Here's how the part is built. I have some questions about the finished solid (model axes, mm). Face numbers are marked on the shaded views. A direction names the side the tool comes from. Give positions to 0.01 mm unless a question says otherwise; leave off trailing zeros. Write each loop counter-clockwise with the first axis right and the second up, starting at its lowest first coordinate (ties: lowest second). Pieces come first, ordered by that corner, then holes. Notation, with made-up numbers: (56.5, 49.5) -> (72.5, 49.5) arc R23 cw to (72.5, 60.5) -> close; hole circle Ø5 at (88, 48.5). An arc over 180 degrees is marked (long way). Use one line per item in the form item = value.
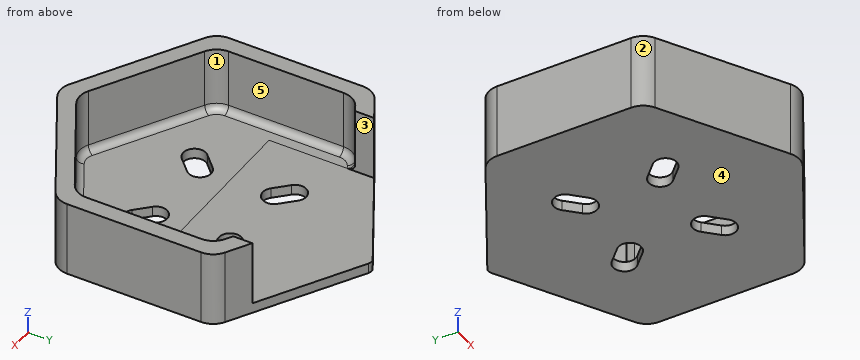
```python
from build123d import *

# Parameters (mm, degrees)
F1_DEPTH = 1.5
F2_DEPTH = 11
F4_W     = 30
F4_H     = 11.070783
F5_DEPTH = 26
F6_R     = 3
F7_R     = 1


with BuildPart() as f1:
    # F0 (on Top) → F1 (new body)
    with BuildSketch(Plane.XY):
        Polygon((0, -20.207259), (17.5, -10.10363), (17.5, 10.10363), (0, 20.207259), (-17.5, 10.10363), (-17.5, -10.10363), align=None)
        with BuildLine():
            ThreePointArc((-6.151829, -8.485281), (-8.485281, -8.485281), (-8.485281, -6.151829))
            Line((-8.485281, -6.151829), (-6.576093, -4.242641))
            ThreePointArc((-6.576093, -4.242641), (-4.242641, -4.242641), (-4.242641, -6.576093))
            Line((-4.242641, -6.576093), (-6.151829, -8.485281))
        make_face(mode=Mode.SUBTRACT)
        with BuildLine():
            ThreePointArc((8.485281, -6.151829), (8.485281, -8.485281), (6.151829, -8.485281))
            Line((6.151829, -8.485281), (4.242641, -6.576093))
            ThreePointArc((4.242641, -6.576093), (4.242641, -4.242641), (6.576093, -4.242641))
            Line((6.576093, -4.242641), (8.485281, -6.151829))
        make_face(mode=Mode.SUBTRACT)
        with BuildLine():
            ThreePointArc((-8.485281, 6.151829), (-8.485281, 8.485281), (-6.151829, 8.485281))
            Line((-6.151829, 8.485281), (-4.242641, 6.576093))
            ThreePointArc((-4.242641, 6.576093), (-4.242641, 4.242641), (-6.576093, 4.242641))
            Line((-6.576093, 4.242641), (-8.485281, 6.151829))
        make_face(mode=Mode.SUBTRACT)
        with BuildLine():
            Line((4.242641, 6.576093), (6.151829, 8.485281))
            ThreePointArc((6.151829, 8.485281), (8.485281, 8.485281), (8.485281, 6.151829))
            Line((8.485281, 6.151829), (6.576093, 4.242641))
            ThreePointArc((6.576093, 4.242641), (4.242641, 4.242641), (4.242641, 6.576093))
        make_face(mode=Mode.SUBTRACT)
    extrude(amount=F1_DEPTH)

    # F0 (on Top) → F2 (join)
    with BuildSketch(Plane.XY):
        Polygon((-19.9, 11.48927), (-19.9, -11.48927), (0, -22.978541), (19.9, -11.48927), (19.9, 11.48927), (0, 22.978541), align=None)
        Polygon((17.5, 10.10363), (17.5, -10.10363), (0, -20.207259), (-17.5, -10.10363), (-17.5, 10.10363), (0, 20.207259), align=None, mode=Mode.SUBTRACT)
    extrude(amount=F2_DEPTH)

    # F4 (on offset) → F5 (cut)
    with BuildSketch(Plane.XZ.offset(-25)):
        with Locations((0, 7.035391)):
            Rectangle(F4_W, F4_H)
    extrude(amount=F5_DEPTH, mode=Mode.SUBTRACT)

    # F6
    f6_edges = [f1.edges().sort_by_distance(p)[0] for p in [
        (19.9, 11.48927, 5.5),
        (-19.9, 11.48927, 5.5),
        (-19.9, -11.48927, 5.5),
        (0, -22.978541, 5.5),
        (19.9, -11.48927, 5.5),
        (17.5, 10.10363, 6.25),
        (17.5, -10.10363, 6.25),
        (0, -20.207259, 6.25),
        (-17.5, -10.10363, 6.25),
        (-17.5, 10.10363, 6.25),
    ]]
    fillet(f6_edges, radius=F6_R)

    # F7
    f7_edges = [f1.edges().sort_by_distance(p)[0] for p in [
        (-15.5, 11.25833, 1.5),
        (0, 22.978541, 0.75),
    ]]
    fillet(f7_edges, radius=F7_R)


solid = f1.part
```
Q1. I want a section at D-D, the plane x = -5. Count the separate pieces of the cut face and the enclosed holes in it, and give its area (3 significant figures).
Result set:
separate_pieces = 3
enclosed_holes = 0
area = 76.3 mm2
Q2. Will these pins go through, and if not, where does the flat tip stop? pin 1 Ø6 at (x, z) = (0, 7) entering from +Y; pin 2 Ø14.5 at (x, y) = (5, 1) entering from +Z; pin 3 Ø1.2 at (y, z) = (12.5, 4) entering from +X.
Result set:
pin_1 = -18.48
pin_2 = 1.5
pin_3 = 19
Q3. I want a section at B-B, the plane z = 1. Write out the boundary of the cut face in (x, y), and give its area (3 significant figures).
Result set:
outline = (-19.9, -9.76) arc R3 ccw to (-18.4, -12.36) -> (-1.5, -22.11) arc R3 ccw to (1.5, -22.11) -> (18.4, -12.36) arc R3 ccw to (19.9, -9.76) -> (19.9, 9.76) arc R3 ccw to (18.4, 12.36) -> (0.5, 22.69) arc R1 ccw to (-0.5, 22.69) -> (-18.4, 12.36) arc R3 ccw to (-19.9, 9.76) -> close; hole (-8.49, -6.15) arc R1.65 ccw to (-6.15, -8.49) -> (-4.24, -6.58) arc R1.65 ccw to (-6.58, -4.24) -> close; hole (-8.49, 6.15) -> (-6.58, 4.24) arc R1.65 ccw to (-4.24, 6.58) -> (-6.15, 8.49) arc R1.65 ccw to start; hole (4.24, -6.58) -> (6.15, -8.49) arc R1.65 ccw to (8.49, -6.15) -> (6.58, -4.24) arc R1.65 ccw to start; hole (4.24, 6.58) arc R1.65 ccw to (6.58, 4.24) -> (8.49, 6.15) arc R1.65 ccw to (6.15, 8.49) -> close
area = 1,300 mm2
Q4. If I drill on line 1 along X through (y, z) = (-4, 6.5); line 2 along Y through (x, z) = (7.5, 0.75); line 3 along Z through (x, y) = (-11, -3.5), over which ranges is the centre line in solid material (lowest first)? Write a range as from..to.
Result set:
line_1 = -19.9..-17.5, 17.5..19.9
line_2 = -18.65..-8.96, -5.17..5.17, 8.96..18.65
line_3 = 0..1.5
Q5. I want a section at A-A, the plane z = 9. Write out the boundary of the cut face in (x, y), and give its area (3 significant figures).
Result set:
outline = (-19.9, -9.76) arc R3 ccw to (-18.4, -12.36) -> (-1.5, -22.11) arc R3 ccw to (1.5, -22.11) -> (18.4, -12.36) arc R3 ccw to (19.9, -9.76) -> (19.9, 9.76) arc R3 ccw to (18.4, 12.36) -> (15, 14.32) -> (15, 11.55) -> (16, 10.97) arc R3 cw to (17.5, 8.37) -> (17.5, -8.37) arc R3 cw to (16, -10.97) -> (1.5, -19.34) arc R3 cw to (-1.5, -19.34) -> (-16, -10.97) arc R3 cw to (-17.5, -8.37) -> (-17.5, 8.37) arc R3 cw to (-16, 10.97) -> (-15, 11.55) -> (-15, 14.32) -> (-18.4, 12.36) arc R3 ccw to (-19.9, 9.76) -> close
area = 228 mm2
Q6. I want a section at C-C, the plane y = 13.5. Write out the boundary of the cut face in (x, z).
Result set:
outline = (-16.42, 0) -> (16.42, 0) -> (16.42, 11) -> (15, 11) -> (15, 1.5) -> (-15, 1.5) -> (-15, 11) -> (-16.42, 11) -> close
Q7. Which directions (+Z, -Z, +X, -X, +Y, -Y) give clear straight access to the entire face, cutting with the end or side of a thin tool? Please do the marked faces 4 and 5.
Result set:
face_4 = -Z, +X, -X, +Y, -Y
face_5 = +Z
Q8. If we mould it in two halves opening along Y, with no side actions, what happens to the marked faces 1, 2 and 3? For each: +Y half, -Y half, draft (parallel to the pull), parting line (faces both ways), or undercut.
Result set:
face_1 = undercut
face_2 = -Y half
face_3 = draft
